Autodesk Inventor part; units mm, degrees
ref_plane "YZ Plane" through (0, 0, 0) normal (1, 0, 0) x (0, 1, 0)
ref_plane "XZ Plane" through (0, 0, 0) normal (0, 1, 0) x (-1, 0, 0)
ref_plane "XY Plane" through (0, 0, 0) normal (0, 0, 1) x (1, 0, 0)
sketch "Sketch1" plane through (0, 0, 0) normal (0, 0, 1) x (1, 0, 0)
  line L0 (0, 8.7149) -> (0, -8.7149) construction
  line L1 (-12.4402, 0) -> (12.4402, 0) construction
  line L2 (-30, 20) -> (30, 20)
  line L3 (30, 20) -> (30, -20)
  line L4 (30, -20) -> (-30, -20)
  line L5 (-30, -20) -> (-30, 20)
  line L6 (-6, 1.25) -> (-2, 1.25)
  line L7 (-2, 1.25) -> (-2, -1.25)
  line L8 (-2, -1.25) -> (-6, -1.25)
  line L9 (-6, -1.25) -> (-6, 1.25)
  line L10 (2, 1.25) -> (6, 1.25)
  line L11 (6, 1.25) -> (6, -1.25)
  line L12 (6, -1.25) -> (2, -1.25)
  line L13 (2, -1.25) -> (2, 1.25)
  point P0 (0, 0)
  point P1 (0, 0)
  dimension "d0" = 4
  dimension "d1" = 4
  dimension "d2" = 4
  dimension "d3" = 2.5
  dimension "d4" = 40
  dimension "d5" = 60
extrude "Extrusion1" add sketch "Sketch1" along normal mid plane 2.5
properties part number "pitahaya3"
Check sheet for the modelled part. Datum: model origin and axes. Units: mm. A direction names the side the tool comes from. Give positions to 0.01 mm unless a question says otherwise; leave off trailing zeros. Answer as a JSON object with one key per item and string values. Group by question number.
Q1. Access from +Z, -Z, +X, -X, +Y, -Y to the whole of each face (thin tool, end or side, straight path). Record for faces 1 (the flat face through (6, 0, 0)), 2 (the flat face through (0, 0, 1.25)).
Q2. Material ranges on line 1 along Y through (x, z) = (-5, 0.25), recorded low to high. Write a range as [from, to].
Q3. Release check for a two-part mould opening along Y. For faces 3 (the flat face through (4, -1.25, 0)), 4 (the flat face through (30, 0, 0)), 5 (the flat face through (0, -20, 0)) record: released by +Y, released by -Y, zero draft, split by the parting line, or undercut.
Evaluation:
{
 "1": {"face 1": "+Z, -Z", "face 2": "+Z, +X, -X, +Y, -Y"},
 "2": {"line 1": "y = [-20, -1.25], [1.25, 20]"},
 "3": {"face 3": "undercut", "face 4": "zero draft", "face 5": "released by -Y"}
}
